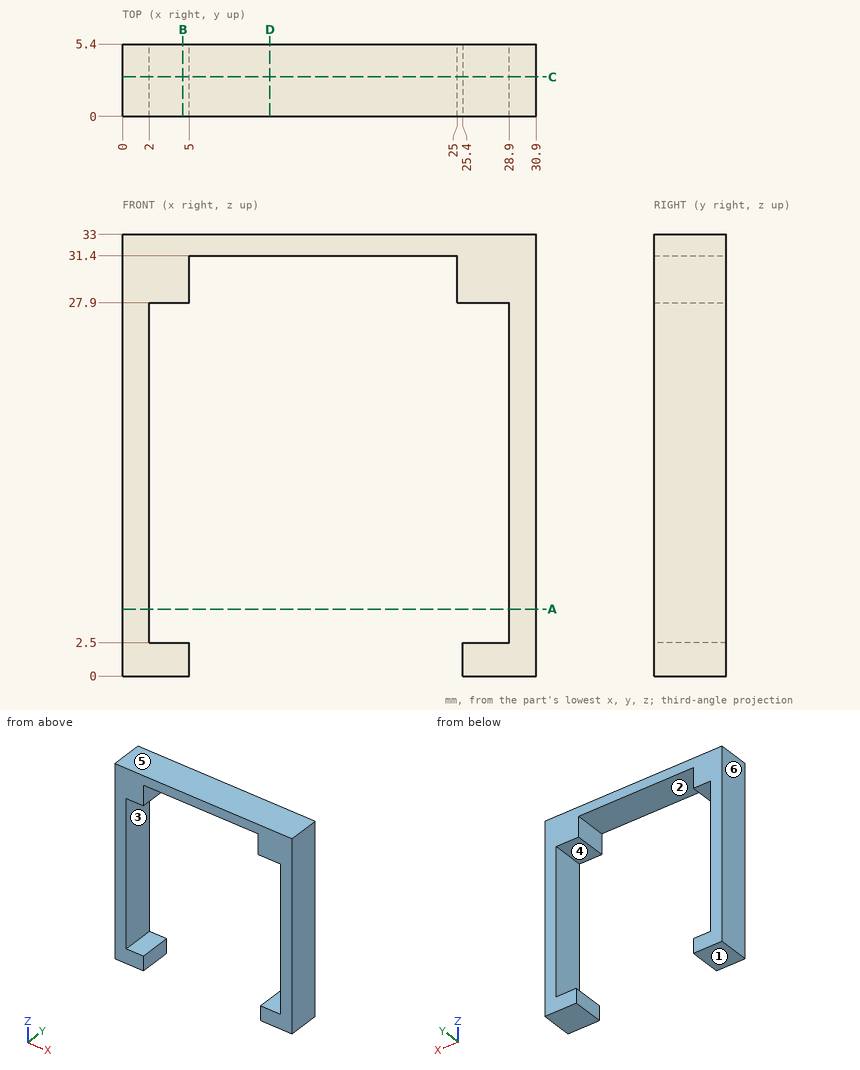
Geometry: see drawing. Coordinates: mm, zero at the bounding-box minimum. A direction names the side the tool comes from. Coordinates: 2 decimals unless noted, no trailing zeros. Write each loop counter-clockwise with the first axis right and the second up, starting at its lowest first coordinate (ties: lowest second). Pieces come first, ordered by that corner, then holes. Notation, with made-up numbers: M -11,32 L 24,32 A21 cw 24,44 Z; hole C 56.25,87.25 d6. An arc over 180 degrees is marked long. Use CSV: the item, a comma, the result in double quotes. Start each with the question number.
1. Cut plane D-D on x = 11. Return the cut outline in (y, z), plus the area to 3 significant figures.
2. Ray query, probe 1 along X at (y, z) = (3.55, 23); probe 2 along X at (y, z) = (5.1, 29); probe 3 along Z at (x, y) = (27, 1.95). Return the intervals inside material, ascending.
3. Cut plane C-C on y = 2.95. Return the cut outline in (x, z).
4. Mould query, pull axis X, two halves, no side actions, for the marked faces 4, 5 and 6. Classes: pulls with the +X half, pulls with the -X half, needs draft (parallel to the pull), parting line crosses it, or undercut.
5. First-contact query: P1, Ø1.6, axis at x = 19, y = 3.5, coming from the -Z side. Flat tip, straight axial feed; report the tip coordinate or a pass-through.
6. Cut plane B-B on x = 4.5. Return the cut outline in (y, z).
7. Reachability of the marked faces 1, 2 and 3 from +Z, -Z, +X, -X, +Y, -Y: full face, straight path, thin tool, end or side. Return the list, or none.
8. Cut plane A-A on z = 5. Return the cut outline in (x, y), plus the area to 3 significant figures.
Entries:
1,outline,"M 0,31.4 L 5.4,31.4 L 5.4,33 L 0,33 Z"
1,area,"8.64 mm²"
2,probe 1,"0 to 2, 28.9 to 30.9"
2,probe 2,"0 to 5, 25 to 30.9"
2,probe 3,"0 to 2.5, 27.9 to 33"
3,outline,"M 0,0 L 5,0 L 5,2.5 L 2,2.5 L 2,27.9 L 5,27.9 L 5,31.4 L 25,31.4 L 25,27.9 L 28.9,27.9 L 28.9,2.5 L 25.4,2.5 L 25.4,0 L 30.9,0 L 30.9,33 L 0,33 Z"
4,face 4,"undercut"
4,face 5,"needs draft"
4,face 6,"pulls with the -X half"
5,P1,"z = 31.4"
6,outline,"M 0,0 L 5.4,0 L 5.4,2.5 L 0,2.5 Z; M 0,27.9 L 5.4,27.9 L 5.4,33 L 0,33 Z"
7,face 1,"-Z, +X, -X, +Y, -Y"
7,face 2,"-Z, +Y, -Y"
7,face 3,"+Y, -Y"
8,outline,"M 0,0 L 2,0 L 2,5.4 L 0,5.4 Z; M 28.9,0 L 30.9,0 L 30.9,5.4 L 28.9,5.4 Z"
8,area,"21.6 mm²"
